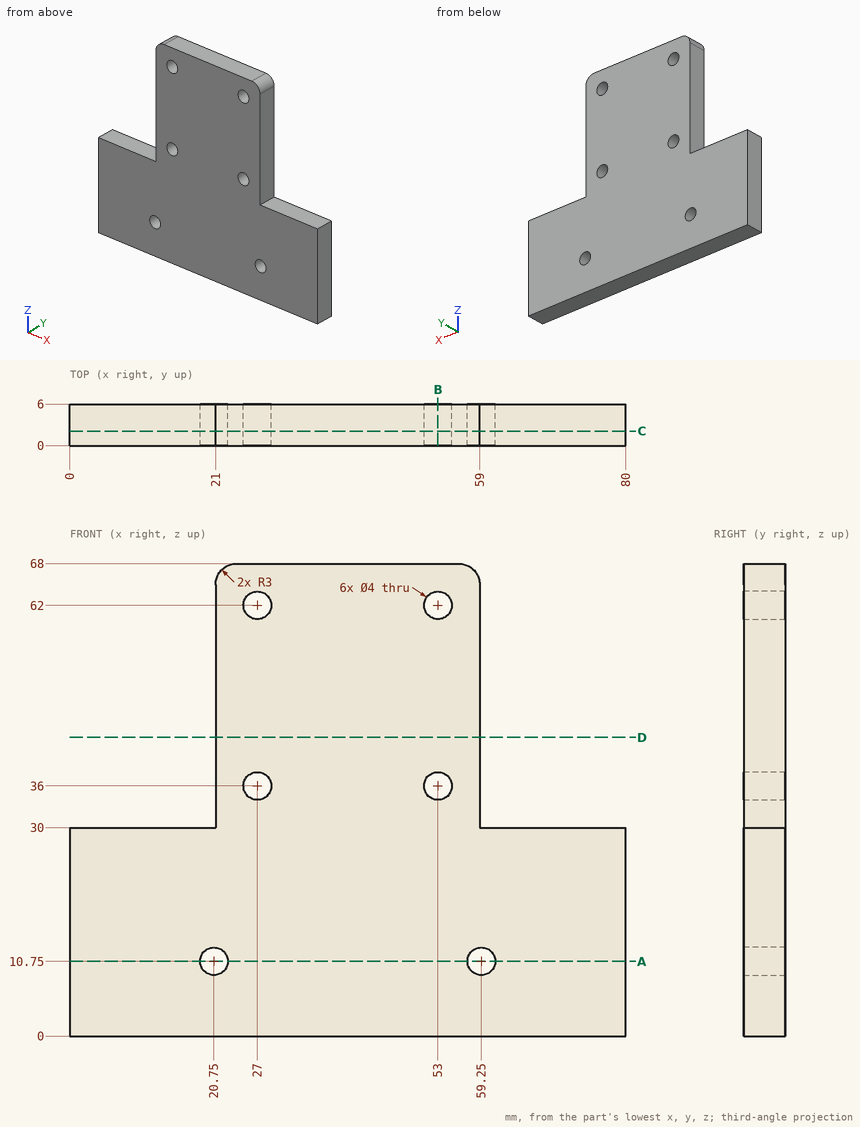
Verification items for this drawing (mm, ordinates from the low corner). Coordinates: 2 decimals unless noted, no trailing zeros. Order: outer loops, then holes, each group sorted by start corner. A loop starts at its lowest first (then second) coordinate and runs counter-clockwise, first axis right, second up. Notation, with made-up numbers: (55, 36) - (108, 36) arc R22 cw to (108, 53) - close; hole circle Ø5 at (15.5, -2). An arc over 180 degrees is marked (long way). Answer as a JSON object with one key per item and string values. Group by question number.
Item 1: Depth check by flat-ended pin: pin 1 Ø3 at (x, y) = (70, 2.5) entering from +Z; pin 2 Ø3 at (y, z) = (2, 37.5) entering from +X; pin 3 Ø2.5 at (x, z) = (27, 62) entering from -Y. Enter the tip coordinate at first touch or a pass-through.
Item 2: Sectioned sample at D-D, the plane z = 43. Record the cut outline in (x, y), and give its area (3 significant figures).
Item 3: Sectioned sample at C-C, the plane y = 2.1. Record the cut outline in (x, z), and give its area (3 significant figures).
Item 4: Scan lines: probe 1 along X at (y, z) = (2.05, 62); probe 2 along X at (y, z) = (2.45, 10.75); probe 3 along X at (y, z) = (5.6, 58.5). Record each from-to range of solid material in increasing order.
Item 5: Sectioned sample at B-B, the plane x = 53. Record the cut outline in (y, z), and give its area (3 significant figures).
Item 6: Sectioned sample at A-A, the plane z = 10.75. Record the cut outline in (x, y).
Resolved:
{
 "1": {"pin 1": "z = 30", "pin 2": "x = 59", "pin 3": "through"},
 "2": {"outline": "(21, 0) - (59, 0) - (59, 6) - (21, 6) - close", "area": "228 mm^2"},
 "3": {"outline": "(0, 0) - (80, 0) - (80, 30) - (59, 30) - (59, 65) arc R3 ccw to (56, 68) - (24, 68) arc R3 ccw to (21, 65) - (21, 30) - (0, 30) - close; hole circle Ø4 at (20.75, 10.75); hole circle Ø4 at (27, 36); hole circle Ø4 at (27, 62); hole circle Ø4 at (53, 36); hole circle Ø4 at (53, 62); hole circle Ø4 at (59.25, 10.75)", "area": "3,760 mm^2"},
 "4": {"probe 1": "21 to 25, 29 to 51, 55 to 59", "probe 2": "0 to 18.75, 22.75 to 57.25, 61.25 to 80", "probe 3": "21 to 59"},
 "5": {"outline": "(0, 0) - (6, 0) - (6, 34) - (0, 34) - close; (0, 38) - (6, 38) - (6, 60) - (0, 60) - close; (0, 64) - (6, 64) - (6, 68) - (0, 68) - close", "area": "360 mm^2"},
 "6": {"outline": "(0, 0) - (18.75, 0) - (18.75, 6) - (0, 6) - close; (22.75, 0) - (57.25, 0) - (57.25, 6) - (22.75, 6) - close; (61.25, 0) - (80, 0) - (80, 6) - (61.25, 6) - close"}
}
